For this review, use the dimensioned drawing (mm, ordinates from the lowest corner) and the shaded views. Give positions to 0.01 mm unless a question says otherwise; leave off trailing zeros. Order: outer loops, then holes, each group sorted by start corner. A loop starts at its lowest first (then second) coordinate and runs counter-clockwise, first axis right, second up. Notation, with made-up numbers: (15, -14) - (37, -14) arc R5 cw to (37, -8) - close; hole circle Ø6 at (62, 21). An arc over 180 degrees is marked (long way). Use a Markdown table: item, result. Add a question column.
1) We need section B-B on y = 11.5. Write out the cut boundary in (x, z), then the cut area to 3 significant figures.
2) Wall thickness on L1, parallel to X at y = 16.5, z = 357; L2, parallel to Z at x = 261, y = 6; L3, parallel to Z at x = 609.5, y = 33: over which ranges is each line inside the solid? List them lowest first.
3) We need section A-A on z = 284. Write out the cut boundary in (x, y).
4) Clearance check with a flat-ended pin moving along its axis: P1, Ø20, axis at x = 271, y = 19.5, coming from the -Z side. State where the tip first meets the part, or that it passes through.
5) We need section C-C on x = 257. Write out the cut boundary in (y, z).
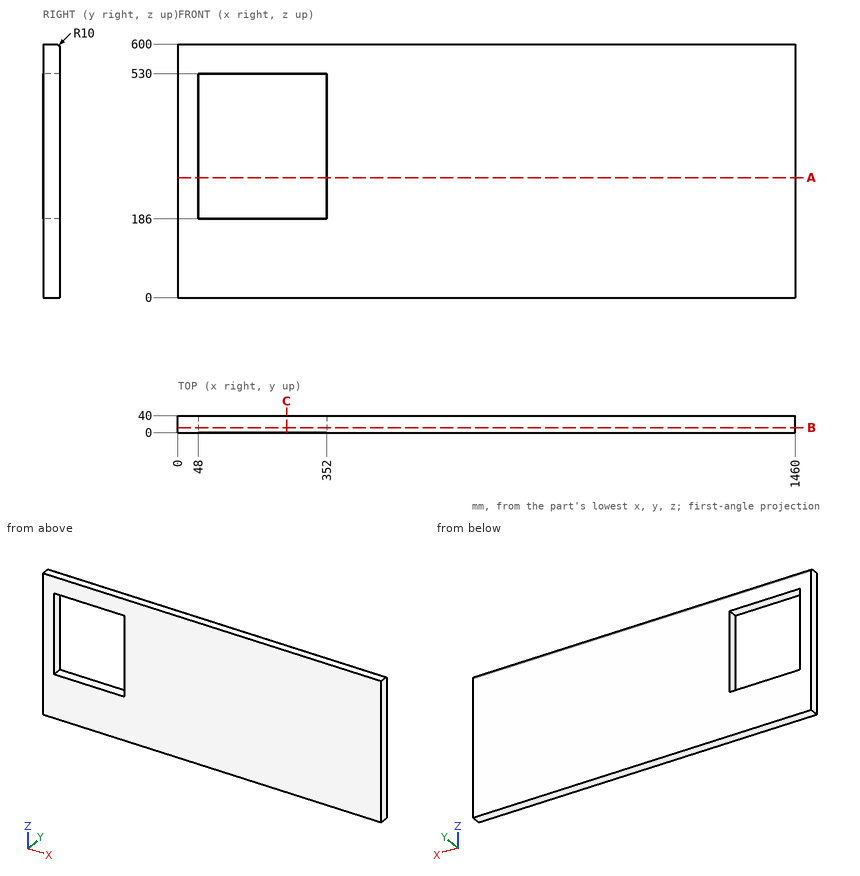
Checked values:
| question | item | result |
|---|---|---|
| 1 | outline | (0, 0) - (1460, 0) - (1460, 600) - (0, 600) - close; hole (48, 186) - (352, 186) - (352, 530) - (48, 530) - close |
| 1 | area | 771,000 mm² |
| 2 | L1 | 0 to 48, 352 to 1460 |
| 2 | L2 | 0 to 186, 530 to 600 |
| 2 | L3 | 0 to 599.54 |
| 3 | outline | (0, 0) - (48, 0) - (48, 40) - (0, 40) - close; (352, 0) - (1460, 0) - (1460, 40) - (352, 40) - close |
| 4 | P1 | z = 0 |
| 5 | outline | (0, 0) - (40, 0) - (40, 186) - (0, 186) - close; (0, 530) - (40, 530) - (40, 590) arc R10 ccw to (30, 600) - (0, 600) - close |
